Autodesk Inventor part; units mm, degrees
ref_plane "YZ Plane" through (0, 0, 0) normal (1, 0, 0) x (0, 1, 0)
ref_plane "XZ Plane" through (0, 0, 0) normal (0, 1, 0) x (-1, 0, 0)
sketch "Sketch1" plane through (0, 0, 0) normal (0, 1, 0) x (-1, 0, 0)
  circle A0 centre (0, 0) radius 9.5
  circle A1 centre (0, 0) radius 7
  circle A2 centre (0, 0) radius 3
  dimension "d0" = 19
  dimension "d1" = 14
  dimension "d6" = 6
extrude "Extrusion1" add sketch "Sketch1" along normal blind 37 contours A0
extrude "Extrusion2" add sketch "Sketch1" along normal blind 3 contours A1
ref_plane "Work Plane1" through (9.5, 37, 0) normal (1, 0, 0) x (0, 1, 0)
sketch "Sketch2" plane through (9.5, 37, 0) normal (1, 0, 0) x (0, 1, 0)
  circle A0 centre (-11.5, 0) radius 5.5
  line L0 (0, -9.5) -> (0, 9.5)
  point P0 (-37, 0)
  point P1 (-6, 0)
  point P2 (0, 0)
  dimension "d7" = 11
  dimension "d9" = 6
extrude "Extrusion3" cut sketch "Sketch2" against normal through all
chamfer "Chamfer2" distance 13.75 distance2 2.5 1 edges at (7, 3, 0) measured on face at (3.14, 21.6954, -6.2562)
properties part number "Mocowanie_do_wieszaka_w_kuchni"
Can you work these out from the model? Positions are in its coordinate system, mm. A direction names the side the tool comes from. Coordinates: 2 decimals unless noted, no trailing zeros. Loops run counter-clockwise (first coordinate to the right, second up) from the corner with the lowest first, then second, coordinate; pieces in that order, holes last. Notation, with made-up numbers: (36, -27) - (72, -27) arc R16 ccw to (72, -2) - close; hole circle Ø10 at (77, 75). An arc over 180 degrees is marked (long way). Answer as CSV lines item,"result". Start each with the question number.
1) Suppose I cut it at C-C (y = 29.5). Please give me the cut outline in (x, z).
2) Which directions (+Z, -Z, +X, -X, +Y, -Y) give clear straight access to the entire face, cutting with the end or side of a thin tool? Please do faces 5 (the cylindrical face through (-3.763, 26.733, -5.902)), 6 (the flat face through (4, 37, -6)).
3) Suppose I cut it at D-D (y = 25.5). Please give me the cut outline in (x, z).
4) Thinking about a two-plate mould opening in Y: for faces 1 (the flat face through (2.24, 0, 2.24)), 2 (the cylindrical face through (6.95, 30.58, -2.11)), 3 (the cylindrical face through (-6.88, 30.58, -2.11)), 4 (the flat face through (-1, 3, -3)), which applies, pulls with the +Y half, pulls with the -Y half, needs draft (parallel to the pull), parting line crosses it, or undercut?
5) For pin 1 (4 mm diameter, centred on x = 6, y = 13, fed in from +Z); pin 2 (8 mm diameter, centred on y = 11, z = -5.5, fed in from -X); pin 3 (1.5 mm diameter, centred on y = 7.5, z = 5.5, fed in from -X); pin 4 (3.5 mm diameter, centred on x = 0, z = 0, fed in from -Y), each with a flat end and sliding along its axis, tell me the tip position at first contact or that it passes through.
6) I need wall thicknesses on line 1 (Z direction, x = 0, y = 1.75); line 2 (X direction, y = 31.25, z = 0); line 3 (Z direction, x = -4.25, y = 17.5). Which ranges of each line are inside material? Lowest first, please. Write a range as from..to.
7) Suppose I cut it at A-A (x = 0). Please give me the cut outline in (y, z), plus the area to 3 significant figures.
8) Suppose I cut it at B-B (z = 0). Please give me the cut outline in (x, y), plus the area to 3 significant figures.
Check result:
1,outline,"(-8.72, -3.77) arc R9.5 ccw to (8.72, -3.77) - (5.89, -3.77) arc R7 cw to (-5.89, -3.77) - close; (-8.72, 3.77) - (-5.89, 3.77) arc R7 cw to (5.89, 3.77) - (8.72, 3.77) arc R9.5 ccw to start"
2,face 5,"+Y"
2,face 6,"+Z, -Z, +X, -X, +Y"
3,outline,"(-7.75, -5.5) arc R9.5 ccw to (7.75, -5.5) - (4.33, -5.5) arc R7 cw to (-4.33, -5.5) - close; (-7.75, 5.5) - (-4.33, 5.5) arc R7 cw to (4.33, 5.5) - (7.75, 5.5) arc R9.5 ccw to start"
4,face 1,"pulls with the -Y half"
4,face 2,"undercut"
4,face 3,"undercut"
4,face 4,"pulls with the +Y half"
5,pin 1,"stops at z = 8.62"
5,pin 2,"stops at x = -9.38"
5,pin 3,"stops at x = -8.23"
5,pin 4,"passes through"
6,line 1,"z = -9.5..-3, 3..9.5"
6,line 2,"x = -9.5..-7, 7..9.5"
6,line 3,"z = -8.5..-5.56, 5.56..8.5"
7,outline,"(0, -9.5) - (37, -9.5) - (37, -7) - (16.75, -7) - (3, -4.5) - (3, -3) - (0, -3) - close; (0, 3) - (3, 3) - (3, 4.5) - (16.75, 7) - (37, 7) - (37, 9.5) - (0, 9.5) - close"
7,area,"243 mm²"
8,outline,"(-9.5, 0) - (-3, 0) - (-3, 3) - (-4.5, 3) - (-7, 16.75) - (-7, 20) - (-9.5, 20) - close; (-9.5, 31) - (-7, 31) - (-7, 37) - (-9.5, 37) - close; (3, 0) - (9.5, 0) - (9.5, 20) - (7, 20) - (7, 16.75) - (4.5, 3) - (3, 3) - close; (7, 31) - (9.5, 31) - (9.5, 37) - (7, 37) - close"
8,area,"188 mm²"
